Geometry: final body of the model. Coordinates: model frame, mm. Coordinates: 2 decimals unless noted, no trailing zeros. Order: outer loops, then holes, each group sorted by start corner. A loop starts at its lowest first (then second) coordinate and runs counter-clockwise, first axis right, second up. Notation, with made-up numbers: (-14, -26.5) -> (43, -26.5) arc R20 ccw to (43, -19.5) -> close; hole circle Ø10 at (25.25, -11.5). An arc over 180 degrees is marked (long way). Use one line per item in the form item = value.
Autodesk Inventor part; units mm, degrees
ref_plane "YZ Plane" through (0, 0, 0) normal (1, 0, 0) x (0, 1, 0)
ref_plane "XZ Plane" through (0, 0, 0) normal (0, 1, 0) x (-1, 0, 0)
ref_plane "XY Plane" through (0, 0, 0) normal (0, 0, 1) x (1, 0, 0)
sketch "Sketch1" plane through (0, 0, 0) normal (0, 1, 0) x (-1, 0, 0)
  line L0 (69.85, 69.85) -> (-69.85, 69.85)
  line L1 (-69.85, 69.85) -> (-69.85, -69.85)
  line L2 (-69.85, -69.85) -> (69.85, -69.85)
  line L3 (69.85, -69.85) -> (69.85, 69.85)
  line L4 (97.79, 0) -> (-97.79, 0)
  line L5 (0, -97.79) -> (0, 97.79)
  point P0 (0, 0)
  dimension "d0" = 139.7
  dimension "d1" = 139.7
extrude "Extrusion1" add sketch "Sketch1" along normal blind 3.175
sketch "Sketch2" plane through (0, 3.175, 0) normal (0, 1, 0) x (1, 0, 0)
  line L0 (-69.85, 69.85) -> (-69.85, -69.85)
  line L1 (-69.85, -69.85) -> (-69.85, -53.975)
  line L2 (-69.85, -53.975) -> (-53.975, -53.975)
  point P0 (0, 0)
  dimension "d4" = 15.875
  dimension "d5" = 15.875
hole "Hole1" at (-53.975, 3.175, 53.975) direction (0, -1, 0) diameter 5.5118 depth 14.1986 tip angle 118
mirror "Mirror4" about plane through (0, 0, 0) normal (0, 0, 1) of "Hole1"
mirror "Mirror5" about plane through (0, 0, 0) normal (1, 0, 0) of "Hole1", "Mirror4"
equation "\"d0\" = d1"
equation "\"d4\" = d5"
properties part number "CH3-DiffHousingBottom"
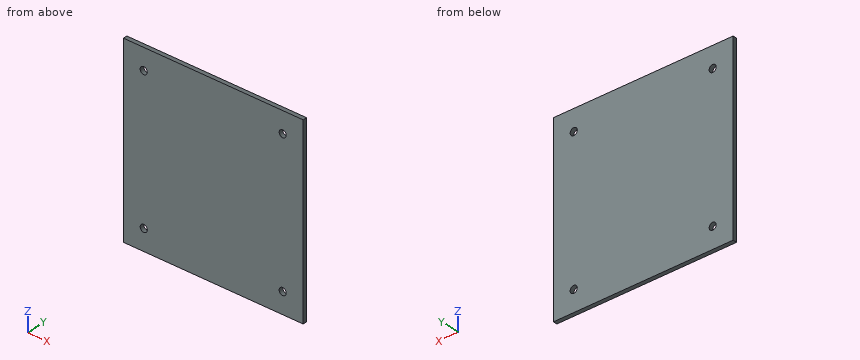
1) Material intervals for probe 1 along X at (y, z) = (2.6, 54); probe 2 along X at (y, z) = (2.5, 53), sorted ascending. Write a range as from..to.
Results found:
probe_1 = -69.85..-56.73, -51.22..51.22, 56.73..69.85
probe_2 = -69.85..-56.55, -51.4..51.4, 56.55..69.85
2) Section A-A, the plane z = -55. Output: boundary loops of the cut face in (x, y) (3 decimals), and give its area (3 significant figures).
Results found:
outline = (-69.85, 0) -> (-56.533, 0) -> (-56.533, 3.175) -> (-69.85, 3.175) -> close; (-51.417, 0) -> (51.417, 0) -> (51.417, 3.175) -> (-51.417, 3.175) -> close; (56.533, 0) -> (69.85, 0) -> (69.85, 3.175) -> (56.533, 3.175) -> close
area = 411 mm2
3) Contact query for a flat-ended pin moving along its axis: P1, Ø3.5, axis at x = 53.975, z = -53.975, coming from the +Y side. Output: stop coordinate, or through.
Results found:
P1 = through
